Can you work these out from the model? Positions are in its coordinate system, mm. Face numbers are marked on the shaded views. Give positions to 0.01 mm unless a question says otherwise; leave off trailing zeros. Write each loop counter-clockwise with the first axis right and the second up, starting at its lowest first coordinate (ties: lowest second). Pieces come first, ordered by that corner, then holes. Notation, with made-up numbers: (-31, 71.5) - (15, 71.5) arc R17 ccw to (15, 99.5) - close; hole circle Ø5 at (9.5, 52). An arc over 180 degrees is marked (long way). Use a Markdown table: item, result. Add a question column.
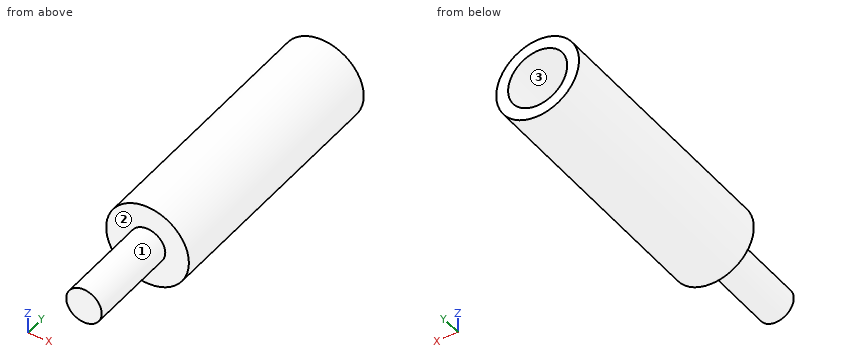
```python
from build123d import *

# Parameters (mm, degrees)
SKETCH1_R           = 3.5
BOSS_EXTRUDE1_DEPTH = 30
SKETCH2_R           = 2.5
CUT_EXTRUDE1_DEPTH  = 20
SKETCH3_R           = 3.5
SKETCH3_R_2         = 1.5
CUT_EXTRUDE4_DEPTH  = 8


with BuildPart() as part:
    # Sketch1 → Boss-Extrude1 (new body)
    with BuildSketch(Plane(origin=(0, 0, 0), x_dir=(1, 0, 0), z_dir=(0, 1, 0))):
        Circle(SKETCH1_R)
    extrude(amount=BOSS_EXTRUDE1_DEPTH)

    # Sketch2 → Cut-Extrude1 (cut)
    with BuildSketch(Plane(origin=(0, 30, 0), x_dir=(1, 0, 0), z_dir=(0, 1, 0))):
        Circle(SKETCH2_R)
    extrude(amount=-CUT_EXTRUDE1_DEPTH, mode=Mode.SUBTRACT)

    # Sketch3 → Cut-Extrude4 (cut)
    with BuildSketch(Plane.XZ):
        Circle(SKETCH3_R)
        Circle(SKETCH3_R_2, mode=Mode.SUBTRACT)
    extrude(amount=-CUT_EXTRUDE4_DEPTH, mode=Mode.SUBTRACT)


solid = part.part
```
Q1. If I drill on probe 1 along X at (y, z) = (24, 0); probe 2 along Y at (x, z) = (-3, -0.5), over which ranges is the centre line in solid material (lowest first)? Write a range as [from, to].
Q2. Suppose I cut it at A-A (x = 0). Please give me the cut outline in (y, z).
Q3. Suppose I cut it at B-B (z = 0). Please give me the cut outline in (x, y).
Q4. Suppose I cut it at C-C (y = 27.5). Please give me the cut outline in (x, z).
Q5. Suppose I cut it at D-D (y = 5). Please give me the cut outline in (x, z).
Q6. I'm going to push flat-ended pins straight in: P1, Ø1.5, axis at x = 0.5, z = -1, coming from the +Y side; P2, Ø2, axis at y = 22.5, z = -2, coming from the -X side; P3, Ø3, axis at y = 26.5, z = -2, coming from the -X side. Where does each tip first touch, or does it pass through?
Q7. If we mould it in two halves opening along X, with no side actions, what happens to the marked faces 1, 2 and 3? For each: released by +X, released by -X, zero draft, split by the parting line, or undercut.
Derived:
| question | item | result |
|---|---|---|
| 1 | probe 1 | [-3.5, -2.5], [2.5, 3.5] |
| 1 | probe 2 | [8, 30] |
| 2 | outline | (0, -1.5) - (8, -1.5) - (8, -3.5) - (30, -3.5) - (30, -2.5) - (10, -2.5) - (10, 2.5) - (30, 2.5) - (30, 3.5) - (8, 3.5) - (8, 1.5) - (0, 1.5) - close |
| 3 | outline | (-3.5, 8) - (-1.5, 8) - (-1.5, 0) - (1.5, 0) - (1.5, 8) - (3.5, 8) - (3.5, 30) - (2.5, 30) - (2.5, 10) - (-2.5, 10) - (-2.5, 30) - (-3.5, 30) - close |
| 4 | outline | circle Ø7 at (0, 0); hole circle Ø5 at (0, 0) |
| 5 | outline | circle Ø3 at (0, 0) |
| 6 | P1 | y = 10 |
| 6 | P2 | x = -3.35 |
| 6 | P3 | x = -3.46 |
| 7 | face 1 | split by the parting line |
| 7 | face 2 | zero draft |
| 7 | face 3 | undercut |
